Autodesk Inventor part; units mm, degrees
ref_plane "YZ Plane" through (0, 0, 0) normal (1, 0, 0) x (0, 1, 0)
ref_plane "XZ Plane" through (0, 0, 0) normal (0, 1, 0) x (-1, 0, 0)
ref_plane "XY Plane" through (0, 0, 0) normal (0, 0, 1) x (1, 0, 0)
sketch "Sketch1" plane through (0, 0, 0) normal (0, 1, 0) x (-1, 0, 0)
  line L0 (12.6289, 26.2657) -> (-103.3711, 26.2657)
  line L1 (-103.3711, 26.2657) -> (-103.3711, -53.7343)
  line L2 (-103.3711, -53.7343) -> (12.6289, -53.7343)
  line L3 (12.6289, -53.7343) -> (12.6289, 26.2657)
  point P0 (0, 0)
  dimension "d0" = 116
  dimension "d1" = 80
extrude "Extrusion1" add sketch "Sketch1" along normal blind 118
sketch "Sketch2" plane through (0, 118, 0) normal (0, 1, 0) x (1, 0, 0)
  circle A0 centre (45.3711, 13.7343) radius 37
  circle A1 centre (45.3711, 13.7343) radius 25
  point P0 (0, 0)
  point P1 (-12.6289, -26.2657)
  dimension "d5" = 74
  dimension "d6" = 50
extrude "Extrusion2" add sketch "Sketch2" along normal blind 1
sketch "Sketch3" plane through (103.3711, 0, -53.7343) normal (0, 0, -1) x (-1, 0, 0)
  line L0 (0, 0) -> (116, 0)
  line L1 (0, 0) -> (33, 0)
  line L2 (33, 0) -> (83, 0)
  line L3 (83, 0) -> (83, 80)
  line L4 (83, 80) -> (33, 80)
  line L5 (33, 80) -> (33, 0)
  point P0 (103.3711, 0)
  dimension "d9" = 33
  dimension "d10" = 50
  dimension "d11" = 80
extrude "Extrusion3" cut sketch "Sketch3" against normal blind 200
sketch "Sketch4" plane through (-12.6289, 0, -53.7343) normal (-1, 0, 0) x (0, 0, 1)
  circle A0 centre (40, 40) radius 40
  line L0 (0, 0) -> (80, 0)
  line L1 (0, 0) -> (0, 118)
  circle A1 centre (40, 40) radius 25
  line L2 (0, 0) -> (0, 118)
  line L3 (0, 118) -> (80, 118)
  line L4 (80, 118) -> (80, 0)
  line L5 (80, 0) -> (0, 0)
  line L6 (0, 0) -> (0, 118)
  point P0 (53.7343, 0)
  point P1 (0, 40)
  point P2 (40, 0)
  point P3 (80, 40)
  dimension "d14" = 80
  dimension "d15" = 50
extrude "Extrusion4" cut sketch "Sketch4" against normal blind 200 contours A1
extrude "Extrusion5" cut sketch "Sketch4" against normal blind 200 contours A0 L0 L1
extrude "Extrusion6" cut sketch "Sketch4" against normal blind 200 contours L4 L0 A0
fillet "Fillet1" radius 10 6 edges at (-12.6289, 0, -13.7343) (-12.6289, 79, -53.7343) (-12.6289, 79, 26.2657) (103.3711, 0, -13.7343) (103.3711, 79, -53.7343) (103.3711, 79, 26.2657)
Here's how the part is built. I have some questions about the finished solid (model axes, mm). A direction names the side the tool comes from. Coordinates: 2 decimals unless noted, no trailing zeros. Loops run counter-clockwise (first coordinate to the right, second up) from the corner with the lowest first, then second, coordinate; pieces in that order, holes last. Notation, with made-up numbers: (-32.5, 84.25) - (24.5, 84.25) arc R21 ccw to (24.5, 112.25) - close; hole circle Ø2 at (68.25, 85). An arc over 180 degrees is marked (long way). Answer as CSV lines item,"result".
Q1. If I drill on L1, parallel to X at y = 34, z = -43.5; L2, parallel to Y at x = 30, z = 0.5; L3, parallel to Y at x = 72.5, z = 6.5, over which ranges is the centre line in solid material (lowest first)? Write a range as [from, to].
Response:
L1,"[-12.62, 20.37], [70.37, 103.36]"
L2,"[80, 118]"
L3,"[5.5, 25.32], [54.68, 119]"
Q2. If we section it at B-B, the plane y = 51: Write out the boundary of the cut face in (x, z).
Response:
outline,"(-12.63, -43.73) arc R10 ccw to (-2.63, -53.73) - (20.37, -53.73) - (20.37, -36.18) - (-12.63, -36.18) - close; (-12.63, 8.72) - (20.37, 8.72) - (20.37, 26.27) - (-2.63, 26.27) arc R10 ccw to (-12.63, 16.27) - close; (70.37, -53.73) - (93.37, -53.73) arc R10 ccw to (103.37, -43.73) - (103.37, -36.18) - (70.37, -36.18) - close; (70.37, 8.72) - (103.37, 8.72) - (103.37, 16.27) arc R10 ccw to (93.37, 26.27) - (70.37, 26.27) - close"
Q3. We'd pull the mould along Y, two halves only. Please class faces 4 (the face through (3.64, 17.82, -2.2)), 5 (the face through (45, 80, -14)), 6 (the face through (70.371, 58.34, 3.48)): pulls with the +Y half, pulls with the -Y half, needs draft (parallel to the pull), parting line crosses it, or undercut.
Response:
face 4,"undercut"
face 5,"pulls with the -Y half"
face 6,"needs draft"
Q4. For pin 1 (25 mm diameter, centred on x = 41.5, z = -14.5, fed in from +Y); pin 2 (6 mm diameter, centred on x = 87.5, z = -11, fed in from -Y); pin 3 (5 mm diameter, centred on x = 90, z = -1, fed in from -Y), each with a flat end and sliding along its axis, tell me the tip position at first contact or that it passes through.
Response:
pin 1,"y = 118"
pin 2,"y = 0"
pin 3,"y = 1.33"
Q5. If we section it at A-A, the plane x = 3: Write out the boundary of the cut face in (y, z), and give its area (3 significant figures).
Response:
outline,"(40, -53.73) - (118, -53.73) - (118, 26.27) - (40, 26.27) arc R40 ccw to start; hole circle Ø50 at (40, -13.73)"
area,"6,790 mm2"
Q6. If we section it at C-C, the plane z = -34: Give the number of separate pieces and of enclosed holes in the cut face, and give its area (3 significant figures).
Response:
separate pieces,"3"
enclosed holes,"0"
area,"7,370 mm2"
Q7. For faces 1 (the face through (20.371, 66, -14)), 2 (the face through (103.371, 75, -13)), 3 (the face through (46, 118, -13)), which set-ups out of +Z, -Z, +X, -X, +Y, -Y let a thin tool reach every point of the face, with its end or its side?
Response:
face 1,"+Z, -Z, -Y"
face 2,"+Z, -Z, +X, +Y, -Y"
face 3,"+Y"
Q8. If we section it at D-D, the plane x = 68.5: Write out the boundary of the cut face in (y, z), and give its area (3 significant figures).
Response:
outline,"(80, -53.73) - (118, -53.73) - (118, -42.61) - (119, -42.61) - (119, -23.22) - (118, -23.22) - (118, -4.24) - (119, -4.24) - (119, 15.15) - (118, 15.15) - (118, 26.27) - (80, 26.27) - close"
area,"3,080 mm2"
